For this review, take the finished solid that the model builds, in its own axes (mm). A direction names the side the tool comes from. Give positions to 0.01 mm unless a question says otherwise; leave off trailing zeros. Write each loop counter-clockwise with the first axis right and the second up, starting at its lowest first coordinate (ties: lowest second). Pieces come first, ordered by that corner, then holes.
Q1. We need section B-B (z = -10). Write out the cut boundary in (x, y).
Q2. We need section A-A (x = -19.05). Write out the cut boundary in (y, z).
Q3. Mouldability with a two-part tool opening along Z and no side actions: class faces 1 (the flat face through (12.7, 9, -1)), 2 (the cylindrical face through (46.88, 15.02, -0.28)), 3 (the flat face through (25, 17, -38.1)) as released by +Z, released by -Z, zero draft, split by the parting line, or undercut.
Q4. Machinability: for faces 4 (the flat face through (40.862, 17.056, -0.267)), 5 (the cylindrical face through (34.97, 19.02, -25.4)), 6 (the flat face through (28.832, 21.126, 0.267)), 7 (the flat face through (-19, 19.05, -1)), 8 (the flat face through (41.8, 9.35, -0.53)), which of the approach directions +Z, -Z, +X, -X, +Y, -Y give a long, thin tool a straight path to every point of the face, cutting with its end or side? Answer none if there is none.
Q5. For line 1 (Z direction, x = -19, y = 27); line 2 (X direction, y = 1.5, z = 12); line 3 (X direction, y = 26.25, z = -19.05), list the stretches that pass through material, from the lowest coordinate up.
Q6. We need section D-D (y = 29). Write out the cut boundary in (x, z).
Q7. Insertion check: P1, Ø20.5, axis at x = -19.05, z = -19.05, coming from the +Y side; P2, Ø14, axis at x = 9, z = 9.5, coming from the -Y side; P3, Ø6, axis at x = -17.5, z = 15.5, coming from the -Y side; P4, Ø1, axis at y = 13.5, z = -9.5, coming from the +X side. Each pin has a flat end and moves straight along its axis. Give the tip position at first contact, or say it passes through.
Q8. We need section C-C (z = -30.5). Write out the cut boundary in (x, y), then the cut area to 3 significant figures.
Autodesk Inventor part; units mm, degrees
ref_plane "YZ Plane" through (0, 0, 0) normal (1, 0, 0) x (0, 1, 0)
ref_plane "XZ Plane" through (0, 0, 0) normal (0, 1, 0) x (-1, 0, 0)
ref_plane "XY Plane" through (0, 0, 0) normal (0, 0, 1) x (1, 0, 0)
sketch "Sketch1" plane through (0, 0, 0) normal (0, 0, 1) x (1, 0, 0)
  line L0 (0, 0) -> (12.7, 0)
  line L1 (12.7, 0) -> (12.7, 19.05)
  line L2 (12.7, 19.05) -> (88.9, -6.35)
  line L3 (88.9, -6.35) -> (88.9, 7.7874)
  line L4 (88.9, 7.7874) -> (19.05, 31.75)
  line L5 (19.05, 31.75) -> (-38.1, 31.75)
  line L6 (-38.1, 31.75) -> (-38.1, 19.05)
  line L7 (-38.1, 19.05) -> (0, 19.05)
  line L8 (0, 19.05) -> (0, 0)
  dimension "d9" = 38.1
  dimension "d10" = 12.7
  dimension "d11" = 19.05
  dimension "d12" = 38.1
  dimension "d13" = 12.7
  dimension "d14" = 127
  dimension "d15" = 57.15
  dimension "d16" = 0.5
extrude "Extrusion1" add sketch "Sketch1" along normal mid plane 76.2
sketch "Sketch2" plane through (-38.1, 31.75, 38.1) normal (0, 1, 0) x (1, 0, 0)
  circle A0 centre (19.05, 19.05) radius 6.35
  circle A1 centre (19.05, 57.15) radius 6.35
  line L0 (57.15, 0) -> (0, 0)
  line L1 (0, 76.2) -> (0, 0)
  point P0 (38.1, 38.1)
  dimension "d19" = 12.7
  dimension "d20" = 12.7
  dimension "d21" = 0
  dimension "d22" = 38.1
  dimension "d23" = 19.05
  dimension "d24" = 19.05
extrude "Extrusion2" cut sketch "Sketch2" against normal through all
sketch "Sketch3" plane through (19.05, 31.75, 38.1) normal (0.3244944, 0.9458876, 0) x (0.9458876, -0.3244944, 0)
  line L0 (19.05, 19.05) -> (19.05, 57.15) construction
  line L1 (12.7, 19.05) -> (12.7, 57.15)
  line L2 (25.4, 57.15) -> (25.4, 19.05)
  arc A0 (12.7, 19.05) -> (25.4, 19.05) centre (19.05, 19.05) ccw
  arc A1 (25.4, 57.15) -> (12.7, 57.15) centre (19.05, 57.15) ccw
  line L3 (-1.8853, 0) -> (78.4335, 0)
  line L4 (0, 76.2) -> (0, 0)
  line L5 (44.45, 25.4) -> (78.4335, 25.4)
  line L6 (78.4335, 76.2) -> (78.4335, 0)
  line L7 (78.4335, 50.8) -> (44.45, 50.8)
  arc A2 (44.45, 50.8) -> (44.45, 25.4) centre (44.45, 38.1) ccw
  point P0 (-7.7165, 38.1)
  point P1 (19.05, 38.1)
  dimension "d27" = 12.7
  dimension "d28" = 38.1
  dimension "d29" = 19.05
  dimension "d30" = 19.05
  dimension "d31" = 25.4
  dimension "d32" = 38.1
  dimension "d33" = 44.45
extrude "Extrusion3" cut sketch "Sketch3" against normal through all
properties part number "HW 7 Part 6" material "Steel, Mild"
Computed:
1. outline: (-38.1, 19.05) - (0, 19.05) - (0, 0) - (12.7, 0) - (12.7, 19.05) - (26.54, 14.44) - (31.06, 27.63) - (19.05, 31.75) - (-38.1, 31.75) - close; (38.59, 10.42) - (49.23, 6.87) - (53.69, 19.87) - (43.08, 23.51) - close
2. outline: (19.05, -38.1) - (31.75, -38.1) - (31.75, -25.4) - (19.05, -25.4) - close; (19.05, -12.7) - (31.75, -12.7) - (31.75, 12.7) - (19.05, 12.7) - close; (19.05, 25.4) - (31.75, 25.4) - (31.75, 38.1) - (19.05, 38.1) - close
3. face 1: zero draft
3. face 2: undercut
3. face 3: released by -Z
4. face 4: +Y
4. face 5: none
4. face 6: -Y
4. face 7: +Z, -Z, -X, -Y
4. face 8: +Z, -Z, -Y
5. line 1: z = -38.1 to -25.4, -12.7 to 12.7, 25.4 to 38.1
5. line 2: x = 0 to 12.7
5. line 3: x = -38.1 to -25.4, -12.7 to 30.59
6. outline: (-38.1, -38.1) - (27.07, -38.1) - (27.07, 38.1) - (-38.1, 38.1) - close; hole circle Ø12.7 at (-19.05, -19.05); hole circle Ø12.7 at (-19.05, 19.05)
7. P1: stops at y = 31.75
7. P2: stops at y = 0
7. P3: stops at y = 19.05
7. P4: stops at x = 51.53
8. outline: (-38.1, 19.05) - (0, 19.05) - (0, 0) - (12.7, 0) - (12.7, 19.05) - (88.9, -6.35) - (88.9, 7.79) - (19.05, 31.75) - (-38.1, 31.75) - close
8. area: 1,990 mm2
